Geometry check sheet. Reference: the model listing, model coordinates, mm. A direction names the side the tool comes from. Round coordinates to 2 decimals unless told otherwise and drop trailing zeros. Loops run counter-clockwise (first coordinate to the right, second up) from the corner with the lowest first, then second, coordinate; pieces in that order, holes last. Notation, with made-up numbers: (-12, -14) -> (10, -14) arc R24 ccw to (10, 16) -> close; hole circle Ø9 at (26.5, -17.5). An arc over 180 degrees is marked (long way). Use a Markdown table: item, result. Add a question column.
Q1. Release check for a two-part mould opening along Z. For faces 1 (the face through (-33.08, -32.39, 100.39)), 2 (the face through (28, 35, 127)), 3 (the face through (86, 1.588, 26)), 4 (the face through (32.39, -33.08, 100.39)) record: released by +Z, released by -Z, zero draft, split by the parting line, or undercut.
Q2. Set-up check for faces 5 (the face through (-1.588, 86, 26)), 6 (the face through (-32.209, 32.894, 108.052)), 7 (the face through (-33.08, -32.39, 115.51)), 8 (the face through (1.588, -86, 26)): record each of +Z, -Z, +X, -X, +Y, -Y from which the full face is reachable in a straight line by a thin tool's end or side.
Q3. Material ranges on L1, parallel to X at y = 91, z = 13.5; L2, parallel to X at y = 0, z = 15.5; L3, parallel to X at y = 0, z = 82 (3 decimals), recorded low to high.
Q4. Sectioned sample at B-B, the plane x = 65. Enter the section's corners in (y, z), then the cut area to 3 significant figures.
Q5. Gauge pin test, flat ends, axial feed: P1, Ø10, axis at y = 90, z = 22, coming from the +X side; P2, Ø6, axis at x = 55, z = 79, coming from the -Y side; P3, Ø1.6, axis at x = 0.5, y = 100.5, coming from the +Z side; P4, Ø1, axis at y = -47, z = 103.5, coming from the +X side. Record the tip position at first contact, or that the pin passes through.
```python
from build123d import *

# Parameters (mm, degrees)
F0_R         = 44.45
F1_DEPTH     = 76.2
F2_R         = 47.625
F2_R_2       = 44.45
F3_DEPTH     = 127
F4_W         = 3.175
F4_H         = 46.0375
F4_H_2       = 3.175
F4_W_2       = 46.0375
F5_DEPTH     = 38.1
F6_W         = 1.5875
F6_H         = 12.7
F8_T2_ANGLE  = 101.902331204
F8_T6_ANGLE  = 101.902331204
F8_S7_R      = 46.0375
F8_T8_DEPTH  = 39
F8_T12_ANGLE = 101.902331204
F8_S13_R     = 46.0375
F8_T14_DEPTH = 39
F8_T18_ANGLE = 101.902331204
F8_S19_R     = 46.0375
F8_T20_DEPTH = 39
F8_T24_ANGLE = 101.902331204
F8_S25_R     = 46.0375
F8_T26_DEPTH = 39
F8_T28_ANGLE = 101.902331204
F8_T32_ANGLE = 101.902331204
F8_S33_R     = 46.0375
F8_T34_DEPTH = 39
F8_T36_ANGLE = 101.902331204
F8_T40_ANGLE = 101.902331204
F8_S41_R     = 46.0375
F8_T42_DEPTH = 39
F8_T44_ANGLE = 101.902331204
F8_T48_ANGLE = 101.902331204
F8_S49_R     = 46.0375
F8_T50_DEPTH = 39
F8_T54_ANGLE = 101.902331204
F8_S55_R     = 46.0375
F8_T56_DEPTH = 39
F9_DEPTH     = 25.4
F11_DEPTH    = 3.175
F13_DEPTH    = 3.175
F15_DEPTH    = 3.175
F17_DEPTH    = 3.175


# Not quite as in the source:
# - a fillet or chamfer that OpenCascade refuses, or shapes differently, is made with other operations: its cross-section is extruded or revolved along the edge and cut away or added


with BuildPart() as f1:
    # F0 (on Top) → F1 (new body)
    with BuildSketch(Plane.XY):
        with BuildLine():
            Line((101.6, 1.5875), (47.598534313, 1.5875))
            ThreePointArc((47.598534313, 1.5875), (33.675960454, 33.675960454), (1.5875, 47.598534313))
            Line((1.5875, 47.598534313), (1.5875, 101.5875968992))
            Line((1.5875, 101.5875968992), (-1.5875, 101.5875968992))
            Line((-1.5875, 101.5875968992), (-1.5875, 47.598534313))
            ThreePointArc((-1.5875, 47.598534313), (-33.675960454, 33.675960454), (-47.598534313, 1.5875))
            Line((-47.598534313, 1.5875), (-101.6, 1.5875))
            Line((-101.6, 1.5875), (-101.6, -1.5875))
            Line((-101.6, -1.5875), (-47.598534313, -1.5875))
            ThreePointArc((-47.598534313, -1.5875), (-33.675960454, -33.675960454), (-1.5875, -47.598534313))
            Line((-1.5875, -47.598534313), (-1.5875, -101.6))
            Line((-1.5875, -101.6), (1.5875, -101.6))
            Line((1.5875, -101.6), (1.5875, -47.598534313))
            ThreePointArc((1.5875, -47.598534313), (33.675960454, -33.675960454), (47.598534313, -1.5875))
            Line((47.598534313, -1.5875), (101.6, -1.5875))
            Line((101.6, -1.5875), (101.6, 1.5875))
        make_face()
        Circle(F0_R, mode=Mode.SUBTRACT)
    extrude(amount=F1_DEPTH)

    # F2 (on Top) → F3 (join)
    with BuildSketch(Plane.XY):
        Circle(F2_R)
        Circle(F2_R_2, mode=Mode.SUBTRACT)
    extrude(amount=F3_DEPTH)

    # F4 (on face) → F5 (cut)
    with BuildSketch(Plane.XY.offset(127)):
        with Locations((0, 24.60625)):
            Rectangle(F4_W, F4_H)
        Rectangle(F4_W, F4_H_2)
        with Locations((-24.60625, 0)):
            Rectangle(F4_W_2, F4_H_2)
        with Locations((0, -24.60625)):
            Rectangle(F4_W, F4_H)
        with Locations((24.60625, 0)):
            Rectangle(F4_W_2, F4_H_2)
    extrude(amount=-F5_DEPTH, mode=Mode.SUBTRACT)

    # F6 (on Right) → F7 (revolve, cut)
    with BuildSketch(Plane.YZ):
        with Locations((-46.83125, 107.95)):
            Rectangle(F6_W, F6_H)
    revolve(axis=Axis((0, 0, 63.5), (0, 0, 1)), mode=Mode.SUBTRACT)

    # F8: chamfer of 2.54 on 12 edges, made by hand

    # F8_s1 → F8_t2 (revolve, cut)
    with BuildSketch(Plane(origin=(0, 0, 0), x_dir=(0, 0, 1), z_dir=(0.1036807735, 0.9946106259, 0))):
        Polygon((127, -45.085), (124.46, -47.625), (127, -47.625), align=None)
    revolve(axis=Axis((0, 0, 127), (0, 0, 1)), revolution_arc=F8_T2_ANGLE, mode=Mode.SUBTRACT)


with BuildPart() as f8_tool4:
    # F8_s5 → F8_t6 (revolve)
    with BuildSketch(Plane(origin=(0, 0, 0), x_dir=(0, 0, 1), z_dir=(0.1036807735, 0.9946106259, 0))):
        Polygon((116.84, -47.625), (114.3, -45.085), (114.3, -47.625), align=None)
    revolve(axis=Axis((0, 0, 114.3), (0, 0, 1)), revolution_arc=F8_T6_ANGLE)

    # F8_s7 → F8_t8 (cut, symmetric)
    with BuildSketch(Plane.XY.offset(115.6)):
        Circle(F8_S7_R)
    extrude(amount=F8_T8_DEPTH, both=True, mode=Mode.SUBTRACT)


with BuildPart() as f1_1:
    add(f1.part)

    # F8_t3: cut F8_tool4
    add(f8_tool4.part, mode=Mode.SUBTRACT)


with BuildPart() as f8_tool10:
    # F8_s11 → F8_t12 (revolve)
    with BuildSketch(Plane(origin=(0, 0, 0), x_dir=(0, 0, 1), z_dir=(0.1036807735, 0.9946106259, 0))):
        Polygon((99.06, -47.625), (101.6, -45.085), (101.6, -47.625), align=None)
    revolve(axis=Axis((0, 0, 101.6), (0, 0, 1)), revolution_arc=F8_T12_ANGLE)

    # F8_s13 → F8_t14 (cut, symmetric)
    with BuildSketch(Plane.XY.offset(100.3)):
        Circle(F8_S13_R)
    extrude(amount=F8_T14_DEPTH, both=True, mode=Mode.SUBTRACT)


with BuildPart() as f1_2:
    add(f1_1.part)

    # F8_t9: cut F8_tool10
    add(f8_tool10.part, mode=Mode.SUBTRACT)


with BuildPart() as f8_tool16:
    # F8_s17 → F8_t18 (revolve)
    with BuildSketch(Plane(origin=(0, 0, 0), x_dir=(0, 0, 1), z_dir=(-0.9946106259, 0.1036807735, 0))):
        Polygon((99.06, -47.625), (101.6, -45.085), (101.6, -47.625), align=None)
    revolve(axis=Axis((0, 0, 101.6), (0, 0, 1)), revolution_arc=F8_T18_ANGLE)

    # F8_s19 → F8_t20 (cut, symmetric)
    with BuildSketch(Plane.XY.offset(100.3)):
        Circle(F8_S19_R)
    extrude(amount=F8_T20_DEPTH, both=True, mode=Mode.SUBTRACT)


with BuildPart() as f1_3:
    add(f1_2.part)

    # F8_t15: cut F8_tool16
    add(f8_tool16.part, mode=Mode.SUBTRACT)


with BuildPart() as f8_tool22:
    # F8_s23 → F8_t24 (revolve)
    with BuildSketch(Plane(origin=(0, 0, 0), x_dir=(0, 0, 1), z_dir=(-0.9946106259, 0.1036807735, 0))):
        Polygon((116.84, -47.625), (114.3, -45.085), (114.3, -47.625), align=None)
    revolve(axis=Axis((0, 0, 114.3), (0, 0, 1)), revolution_arc=F8_T24_ANGLE)

    # F8_s25 → F8_t26 (cut, symmetric)
    with BuildSketch(Plane.XY.offset(115.6)):
        Circle(F8_S25_R)
    extrude(amount=F8_T26_DEPTH, both=True, mode=Mode.SUBTRACT)


with BuildPart() as f1_4:
    add(f1_3.part)

    # F8_t21: cut F8_tool22
    add(f8_tool22.part, mode=Mode.SUBTRACT)

    # F8_s27 → F8_t28 (revolve, cut)
    with BuildSketch(Plane(origin=(0, 0, 0), x_dir=(0, 0, 1), z_dir=(-0.9946106259, 0.1036807735, 0))):
        Polygon((127, -45.085), (124.46, -47.625), (127, -47.625), align=None)
    revolve(axis=Axis((0, 0, 127), (0, 0, 1)), revolution_arc=F8_T28_ANGLE, mode=Mode.SUBTRACT)


with BuildPart() as f8_tool30:
    # F8_s31 → F8_t32 (revolve)
    with BuildSketch(Plane(origin=(0, 0, 0), x_dir=(0, 0, 1), z_dir=(0.9946106259, -0.1036807735, 0))):
        Polygon((116.84, -47.625), (114.3, -45.085), (114.3, -47.625), align=None)
    revolve(axis=Axis((0, 0, 114.3), (0, 0, 1)), revolution_arc=F8_T32_ANGLE)

    # F8_s33 → F8_t34 (cut, symmetric)
    with BuildSketch(Plane.XY.offset(115.6)):
        Circle(F8_S33_R)
    extrude(amount=F8_T34_DEPTH, both=True, mode=Mode.SUBTRACT)


with BuildPart() as f1_5:
    add(f1_4.part)

    # F8_t29: cut F8_tool30
    add(f8_tool30.part, mode=Mode.SUBTRACT)

    # F8_s35 → F8_t36 (revolve, cut)
    with BuildSketch(Plane(origin=(0, 0, 0), x_dir=(0, 0, 1), z_dir=(0.9946106259, -0.1036807735, 0))):
        Polygon((127, -45.085), (124.46, -47.625), (127, -47.625), align=None)
    revolve(axis=Axis((0, 0, 127), (0, 0, 1)), revolution_arc=F8_T36_ANGLE, mode=Mode.SUBTRACT)


with BuildPart() as f8_tool38:
    # F8_s39 → F8_t40 (revolve)
    with BuildSketch(Plane(origin=(0, 0, 0), x_dir=(0, 0, 1), z_dir=(0.9946106259, -0.1036807735, 0))):
        Polygon((99.06, -47.625), (101.6, -45.085), (101.6, -47.625), align=None)
    revolve(axis=Axis((0, 0, 101.6), (0, 0, 1)), revolution_arc=F8_T40_ANGLE)

    # F8_s41 → F8_t42 (cut, symmetric)
    with BuildSketch(Plane.XY.offset(100.3)):
        Circle(F8_S41_R)
    extrude(amount=F8_T42_DEPTH, both=True, mode=Mode.SUBTRACT)


with BuildPart() as f1_6:
    add(f1_5.part)

    # F8_t37: cut F8_tool38
    add(f8_tool38.part, mode=Mode.SUBTRACT)

    # F8_s43 → F8_t44 (revolve, cut)
    with BuildSketch(Plane(origin=(0, 0, 0), x_dir=(0, 0, 1), z_dir=(-0.1036807735, -0.9946106259, 0))):
        Polygon((127, -45.085), (124.46, -47.625), (127, -47.625), align=None)
    revolve(axis=Axis((0, 0, 127), (0, 0, 1)), revolution_arc=F8_T44_ANGLE, mode=Mode.SUBTRACT)


with BuildPart() as f8_tool46:
    # F8_s47 → F8_t48 (revolve)
    with BuildSketch(Plane(origin=(0, 0, 0), x_dir=(0, 0, 1), z_dir=(-0.1036807735, -0.9946106259, 0))):
        Polygon((116.84, -47.625), (114.3, -45.085), (114.3, -47.625), align=None)
    revolve(axis=Axis((0, 0, 114.3), (0, 0, 1)), revolution_arc=F8_T48_ANGLE)

    # F8_s49 → F8_t50 (cut, symmetric)
    with BuildSketch(Plane.XY.offset(115.6)):
        Circle(F8_S49_R)
    extrude(amount=F8_T50_DEPTH, both=True, mode=Mode.SUBTRACT)


with BuildPart() as f1_7:
    add(f1_6.part)

    # F8_t45: cut F8_tool46
    add(f8_tool46.part, mode=Mode.SUBTRACT)


with BuildPart() as f8_tool52:
    # F8_s53 → F8_t54 (revolve)
    with BuildSketch(Plane(origin=(0, 0, 0), x_dir=(0, 0, 1), z_dir=(-0.1036807735, -0.9946106259, 0))):
        Polygon((99.06, -47.625), (101.6, -45.085), (101.6, -47.625), align=None)
    revolve(axis=Axis((0, 0, 101.6), (0, 0, 1)), revolution_arc=F8_T54_ANGLE)

    # F8_s55 → F8_t56 (cut, symmetric)
    with BuildSketch(Plane.XY.offset(100.3)):
        Circle(F8_S55_R)
    extrude(amount=F8_T56_DEPTH, both=True, mode=Mode.SUBTRACT)


with BuildPart() as f1_8:
    add(f1_7.part)

    # F8_t51: cut F8_tool52
    add(f8_tool52.part, mode=Mode.SUBTRACT)

    # F9 (add): a face of the model
    f9_faces = [f1_8.faces().sort_by_distance(p)[0] for p in [
        (0, -98.7264057431, 0),
    ]]
    extrude(f9_faces, amount=F9_DEPTH)

    # F10 (on face) → F11 (join, through all)
    with BuildSketch(Plane(origin=(0, 1.5875, 0), x_dir=(-1, 0, 0), z_dir=(0, 1, 0))):
        Polygon((123.7956061959, 76.2), (101.6, 76.2), (101.6, -25.4), (149.198534313, -25.4), align=None)
    extrude(amount=-F11_DEPTH)

    # F12 (on face) → F13 (join, through all)
    with BuildSketch(Plane.YZ.offset(1.5875)):
        Polygon((101.5875968992, 76.2), (101.5875968992, -25.4), (149.198534313, -25.4), (123.798534313, 76.2), align=None)
    extrude(amount=-F13_DEPTH)

    # F14 (on face) → F15 (join, through all)
    with BuildSketch(Plane.XZ.offset(1.5875)):
        Polygon((123.798534313, 76.2), (101.6, 76.2), (101.6, -25.4), (149.198534313, -25.4), align=None)
    extrude(amount=-F15_DEPTH)

    # F16 (on face) → F17 (join, through all)
    with BuildSketch(Plane(origin=(-1.5875, 0, 0), x_dir=(0, -1, 0), z_dir=(-1, 0, 0))):
        Polygon((123.798534313, 76.2), (101.6, 76.2), (101.6, -25.4), (149.198534313, -25.4), align=None)
    extrude(amount=-F17_DEPTH)


solid = f1_8.part
```
Values:
| question | item | result |
|---|---|---|
| 1 | face 1 | undercut |
| 1 | face 2 | released by +Z |
| 1 | face 3 | zero draft |
| 1 | face 4 | undercut |
| 2 | face 5 | +Z, -Z, -X, +Y |
| 2 | face 6 | -X, +Y |
| 2 | face 7 | -X, -Y |
| 2 | face 8 | +Z, -Z, +X, -Y |
| 3 | L1 | -1.59 to 1.59 |
| 3 | L2 | -138.97 to -44.45, 44.45 to 138.97 |
| 3 | L3 | -47.625 to -44.45, 44.45 to 47.625 |
| 4 | outline | (-1.59, -25.4) -> (1.59, -25.4) -> (1.59, 76.2) -> (-1.59, 76.2) -> close |
| 4 | area | 323 mm^2 |
| 5 | P1 | x = 1.59 |
| 5 | P2 | y = -1.59 |
| 5 | P3 | z = 76.2 |
| 5 | P4 | through |
